Autodesk Inventor part; units mm, degrees
ref_plane "YZ Plane" through (0, 0, 0) normal (1, 0, 0) x (0, 1, 0)
ref_plane "XZ Plane" through (0, 0, 0) normal (0, 1, 0) x (-1, 0, 0)
ref_plane "XY Plane" through (0, 0, 0) normal (0, 0, 1) x (1, 0, 0)
sketch "Sketch1" plane through (0, 0, 0) normal (1, 0, 0) x (0, 1, 0)
  line L0 (0, 0) -> (-2, 0)
  line L1 (-2, 0) -> (-2, -19)
  line L2 (-2, -19) -> (0, -19)
  line L3 (0, -19) -> (0, 0)
  line L4 (0, 0) -> (30, 0)
  line L5 (30, 0) -> (30, 2)
  line L6 (30, 2) -> (0, 2)
  line L7 (0, 2) -> (0, 0)
  line L8 (-2, -19) -> (-32, -19)
  line L9 (-32, -19) -> (-32, -16.849)
  line L10 (-32, -16.849) -> (-2, -16.849)
  line L11 (-2, -16.849) -> (-2, -19)
  line L12 (0, 0) -> (-2, 0)
  line L13 (-2, 0) -> (-2, 2)
  line L14 (-2, 2) -> (0, 2)
  line L15 (0, 2) -> (0, 0)
  point P0 (-2, -16.849)
  dimension "d0" = 2
  dimension "d1" = 19
  dimension "d2" = 30
  dimension "d3" = 2
  dimension "d4" = 30
extrude "Extrusion1" add sketch "Sketch1" along normal blind 30
sketch "Sketch2" plane through (0, -2, 2) normal (0, 0, 1) x (1, 0, 0)
  line L0 (0, 0) -> (30, 0)
  line L1 (0, 0) -> (15, 0)
  line L2 (15, 0) -> (15, 17)
  circle A0 centre (15, 17) radius 3
  point P0 (0, 2)
  dimension "d7" = 17
  dimension "d8" = 6
hole "Hole1" at (15, 15, 2) direction (0, 0, -1) diameter 6 end through all
sketch "Sketch4" plane through (0, -32, -19) normal (0, 0, -1) x (-1, 0, 0)
  line L0 (0, 32) -> (-15, 32)
  line L1 (0, 32) -> (-30, 32)
  line L2 (-15, 32) -> (-15, 13)
  dimension "d25" = 19
hole "Hole3" at (15, -19, -19) direction (0, 0, 1) diameter 4 end through all
sketch "Sketch5" plane through (0, -32, -19) normal (0, -1, 0) x (1, 0, 0)
  line L0 (0, 0) -> (30, 0)
  line L1 (0, 2.151) -> (30, 2.151)
  line L2 (30, 0) -> (0, 0)
  line L3 (0, 0) -> (0, 2.151)
  line L4 (0, 2.151) -> (30, 2.151)
  line L5 (30, 2.151) -> (30, 0)
  point P0 (0, 19)
extrude "Extrusion2" cut sketch "Sketch5" against normal blind 5
thread "Thread1"
properties part number "transversal-2l-stabilizer" material "Aluminum 6061"
For this review, take the finished solid that the model builds, in its own axes (mm). A direction names the side the tool comes from. Round coordinates to 2 decimals unless told otherwise and drop trailing zeros. Write each loop counter-clockwise with the first axis right and the second up, starting at its lowest first coordinate (ties: lowest second). Pieces come first, ordered by that corner, then holes. Notation, with made-up numbers: (53, 40) - (103, 40) arc R27 ccw to (103, 73) - close; hole circle Ø10 at (40.5, 17). An arc over 180 degrees is marked (long way). Write item = value, one per line. Start each with the question number.
1. Wall thickness on L1, parallel to Y at x = 15, z = -18.1; L2, parallel to X at y = -19, z = -17.35; L3, parallel to Y at x = 15, z = 0.75: over which ranges is each line inside the solid? List them lowest first.
2. Draft analysis for pull direction X (two halves, no side actions). For faces 1 (the face through (15, -14, -19)), 2 (the face through (13, -19, -18)), 3 (the face through (30, -1, -8)), 4 (the face through (16.8, 17.4, 1)), state which applies: released by +X, released by -X, zero draft, split by the parting line, or undercut.
3. Consider section B-B on x = 15. State the section outline as (y, z) points.
4. Consider section D-D on y = -19. State the section outline as (x, z) points.
5. Consider section C-C on x = 4.25. State the section outline as (y, z) points.
6. For faces 5 (the face through (11, 14, 2)), 6 (the face through (15, 11, 0)), 7 (the face through (15, -2, -7)), list the 3-axis set-ups (+Z, -Z, +X, -X, +Y, -Y) from which the entire face can be reached by the end or side of a thin tool; tool diameter is ignored.
7. Consider section A-A on y = 15. State the section outline as (x, z) points.
8. For pin 1 Ø9.5 at (x, z) = (7.5, -7.5) entering from +Y; pin 2 Ø1 at (x, z) = (17, -0.5) entering from -Y; pin 3 Ø8 at (x, y) = (15, 15) entering from -Z, all flat-tipped, find the tip position at first contact; note any pin that passes through.
Evaluation:
q1.L1 = -27 to -21, -17 to 0
q1.L2 = 0 to 13, 17 to 30
q1.L3 = -2 to 12, 18 to 30
q2.face_1 = zero draft
q2.face_2 = undercut
q2.face_3 = released by +X
q2.face_4 = undercut
q3.outline = (-27, -19) - (-21, -19) - (-21, -16.85) - (-27, -16.85) - close; (-17, -19) - (0, -19) - (0, 0) - (12, 0) - (12, 2) - (-2, 2) - (-2, -16.85) - (-17, -16.85) - close; (18, 0) - (30, 0) - (30, 2) - (18, 2) - close
q4.outline = (0, -19) - (13, -19) - (13, -16.85) - (0, -16.85) - close; (17, -19) - (30, -19) - (30, -16.85) - (17, -16.85) - close
q5.outline = (-27, -19) - (0, -19) - (0, 0) - (30, 0) - (30, 2) - (-2, 2) - (-2, -16.85) - (-27, -16.85) - close
q6.face_5 = +Z, +X, -X, +Y, -Y
q6.face_6 = -Z, +X, -X, +Y
q6.face_7 = +Z, +X, -X, -Y
q7.outline = (0, 0) - (12, 0) - (12, 2) - (0, 2) - close; (18, 0) - (30, 0) - (30, 2) - (18, 2) - close
q8.pin_1 = 0
q8.pin_2 = -2
q8.pin_3 = 0
